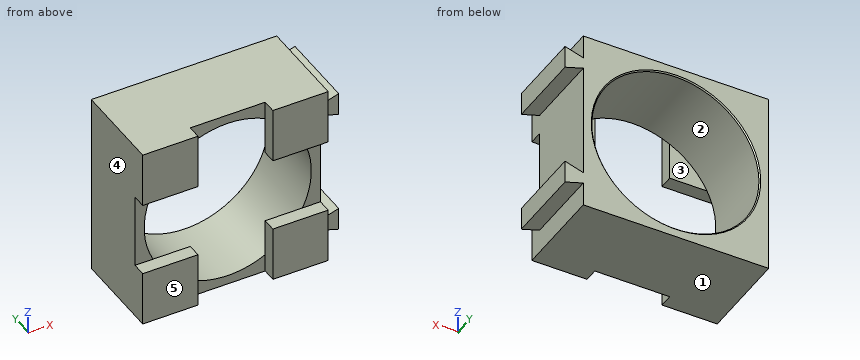
from build123d import *

# Parameters (mm, degrees)
SKETCH1_R              = 9.15
CELL_HOLDER_DEPTH      = 8.5
SKETCH2_W              = 6.05
SKETCH2_H              = 6.05
BOTTOM_BASE_BOSS_DEPTH = 1.5
CHAMFER1_SIZE          = 0.125


with BuildPart() as part:
    # Sketch1 → Cell Holder (new body)
    with BuildSketch(Plane(origin=(0, 0, 0), x_dir=(1, 0, 0), z_dir=(0, 1, 0))):
        Polygon((12.15, 8.15), (12.15, 5.65), (10.15, 6.275), (10.15, -6.275), (12.15, -5.65), (12.15, -8.15), (10.15, -7.525), (10.15, -10.15), (-10.15, -10.15), (-10.15, 10.15), (10.15, 10.15), (10.15, 7.525), align=None)
        with Locations(Location((0, 0, 0), (0, 0, 270))):
            Circle(SKETCH1_R, mode=Mode.SUBTRACT)
    extrude(amount=CELL_HOLDER_DEPTH)

    # Sketch2 → Bottom Base Boss (add)
    with BuildSketch(Plane.XZ):
        with Locations((-7.125, 7.125)):
            Rectangle(SKETCH2_W, SKETCH2_H)
        with Locations((-7.125, -7.125)):
            Rectangle(SKETCH2_W, SKETCH2_H)
        with Locations((7.125, 7.125)):
            Rectangle(SKETCH2_W, SKETCH2_H)
        with Locations((7.125, -7.125)):
            Rectangle(SKETCH2_W, SKETCH2_H)
    extrude(amount=BOTTOM_BASE_BOSS_DEPTH)

    # Chamfer1
    chamfer1_edges = [part.edges().sort_by_distance(p)[0] for p in [
        (0, 8.5, -9.15),
    ]]
    chamfer(chamfer1_edges, length=CHAMFER1_SIZE)


solid = part.part
Model file for the job. Use its own axes, mm. Face numbers are marked on the shaded views. A direction names the side the tool comes from. Coordinates: 2 decimals unless noted, no trailing zeros. Write each loop counter-clockwise with the first axis right and the second up, starting at its lowest first coordinate (ties: lowest second). Pieces come first, ordered by that corner, then holes. Notation, with made-up numbers: (55, 18) - (110, 18) arc R30 cw to (110, 42) - close; hole circle Ø1 at (6.5, 8). An arc over 180 degrees is marked (long way). Write each question's results on one line, items separated by ' | '. Start each with the question number.
1) Flat gauge pins, fed straight in: P1, Ø1.6, axis at x = 11, z = -7.5, coming from the -Y side; P2, Ø1.6, axis at y = -1, z = -6.5, coming from the +X side; P3, Ø1.2, axis at x = -5, z = 6, coming from the +Y side; P4, Ø4, axis at y = 5, z = -5.5, coming from the +X side. Where does each tip first touch, or does it go through?
2) Cut at D-D (y = 1.5). Write the cut outline in (x, z) (3 decimals).
3) Cut at B-B (x = 0). Write the cut outline in (y, z) (3 decimals), then the cut area to 3 significant figures.
4) Cut at C-C (y = -0.75). Write the cut outline in (x, z).
5) Cut at A-A (z = 0). Write the cut outline in (x, y) (3 decimals), then the cut area to 3 significant figures.
6) Mould opens along X. For the marked faces 3, 4 and 5 say: pulls with the +X half, pulls with the -X half, needs draft (parallel to the pull), parting line crosses it, or undercut.
7) Probe line 1 along X through (y, z) = (4.5, 0); line 2 along Z through (x, y) = (4.5, 5.5). List the from-to ranges inside material, lowest first. Write a range as from..to.
8) 3-axis set-ups, long thin cutter, end or side, ignore diameter. For the marked faces 1 and 2: which of +Z, -Z, +X, -X, +Y, -Y reach the whole face in a straight line?
Returned:
1) P1: y = 0 | P2: x = 10.15 | P3: y = 0 | P4: x = 12.15
2) outline: (-10.15, -10.15) - (10.15, -10.15) - (10.15, -7.525) - (12.15, -8.15) - (12.15, -5.65) - (10.15, -6.275) - (10.15, 6.275) - (12.15, 5.65) - (12.15, 8.15) - (10.15, 7.525) - (10.15, 10.15) - (-10.15, 10.15) - close; hole circle Ø18.3 at (0, 0)
3) outline: (0, -10.15) - (8.5, -10.15) - (8.5, -9.275) - (8.375, -9.15) - (0, -9.15) - close; (0, 9.15) - (8.375, 9.15) - (8.5, 9.275) - (8.5, 10.15) - (0, 10.15) - close | area: 17.0 mm^2
4) outline: (-10.15, -10.15) - (-4.1, -10.15) - (-4.1, -4.1) - (-10.15, -4.1) - close; (-10.15, 4.1) - (-4.1, 4.1) - (-4.1, 10.15) - (-10.15, 10.15) - close; (4.1, -10.15) - (10.15, -10.15) - (10.15, -4.1) - (4.1, -4.1) - close; (4.1, 4.1) - (10.15, 4.1) - (10.15, 10.15) - (4.1, 10.15) - close
5) outline: (-10.15, 0) - (-9.15, 0) - (-9.15, 8.375) - (-9.275, 8.5) - (-10.15, 8.5) - close; (9.15, 0) - (10.15, 0) - (10.15, 8.5) - (9.275, 8.5) - (9.15, 8.375) - close | area: 17.0 mm^2
6) face 3: undercut | face 4: pulls with the -X half | face 5: needs draft
7) line 1: -10.15..-9.15, 9.15..10.15 | line 2: -10.15..-7.97, 7.97..10.15
8) face 1: -Z, +X, -X, +Y, -Y | face 2: +Y
